```python
from build123d import *

# Parameters (mm, degrees)
SKETCH1_R               = 50
SKETCH1_R_2             = 10
BOSS_EXTRUDE1_DEPTH     = 3
BOSS_EXTRUDE2_DEPTH     = 2.5
CAVITY2_START           = 0.75
CAVITY2_DEPTH           = 2.25
CAVITY2_START_2         = 1.25
CAVITY2_2_DEPTH         = 1.75
FILLET1_R               = 0.5
FILLET2_R               = 7
CUT_EXTRUDE2_DEPTH      = 76.690157881
CUT_EXTRUDE2_DEPTH_BACK = 76.690157881
SKETCH3_R               = 50
SKETCH3_W               = 41.955661048
SKETCH3_H               = 23.335406012


# Read off the part's stored shape, not the designer's step: Cavity2
with BuildPart() as part:
    # Sketch1 → Boss-Extrude1 (new body)
    with BuildSketch(Plane(origin=(0, 0, 0), x_dir=(1, 0, 0), z_dir=(0, 1, 0))):
        with Locations(Location((0, 0, 0), (0, 0, 270))):
            Circle(SKETCH1_R)
        with Locations(Location((0, 0, 0), (0, 0, 270))):
            Circle(SKETCH1_R_2, mode=Mode.SUBTRACT)
    extrude(amount=BOSS_EXTRUDE1_DEPTH)

    # Sketch2 → Boss-Extrude2 (add, symmetric)
    with BuildSketch(Plane.XY.offset(-25)):
        Polygon((-17.5, 3), (-10.5, 3), (-10.5, 23), (30.5, 23), (30.5, 3), (37.5, 3), (37.5, 30), (-17.5, 30), align=None)
    extrude(amount=BOSS_EXTRUDE2_DEPTH, both=True)

    # Cavity2 outline → Cavity2 (cut)
    with BuildSketch(Plane(origin=(0, 0, 0), x_dir=(1, 0, 0), z_dir=(0, 1, 0)).offset(CAVITY2_START)):
        with BuildLine():
            ThreePointArc((-9.944972826, -1.047623734), (-10, 0), (-9.944972826, 1.047623734))
            ThreePointArc((-9.944972826, 1.047623734), (-10.619281402, 1.655282378), (-11.5, 1.875))
            Line((-11.5, 1.875), (-11.5, 8.875))
            Line((-11.5, 8.875), (-24.1, 8.875))
            Line((-24.1, 8.875), (-24.1, -8.875))
            Line((-24.1, -8.875), (-11.5, -8.875))
            Line((-11.5, -8.875), (-11.5, -1.875))
            ThreePointArc((-11.5, -1.875), (-10.619281402, -1.655282378), (-9.944972826, -1.047623734))
        make_face()
    extrude(amount=CAVITY2_DEPTH, mode=Mode.SUBTRACT)

    # Cavity2 2 outline → Cavity2 2 (cut)
    with BuildSketch(Plane(origin=(0, 0, 0), x_dir=(1, 0, 0), z_dir=(0, 1, 0)).offset(CAVITY2_START_2)):
        with BuildLine():
            ThreePointArc((-11.5, 1.875), (-10.619281402, 1.655282378), (-9.944972826, 1.047623734))
            ThreePointArc((-9.944972826, 1.047623734), (-8.262249735, 5.633402996), (-4.608077148, 8.875))
            Line((-4.608077148, 8.875), (-11.5, 8.875))
            Line((-11.5, 8.875), (-11.5, 1.875))
        make_face()
        with BuildLine():
            ThreePointArc((-4.608077148, -8.875), (-8.262249735, -5.633402996), (-9.944972826, -1.047623734))
            ThreePointArc((-9.944972826, -1.047623734), (-10.619281402, -1.655282378), (-11.5, -1.875))
            Line((-11.5, -1.875), (-11.5, -8.875))
            Line((-11.5, -8.875), (-4.608077148, -8.875))
        make_face()
        with BuildLine():
            Line((-24.1, -4.625), (-24.1, 4.625))
            ThreePointArc((-24.1, 4.625), (-26.35, 0), (-24.1, -4.625))
        make_face()
    extrude(amount=CAVITY2_2_DEPTH, mode=Mode.SUBTRACT)

    # Fillet1
    fillet1_edges = [part.edges().sort_by_distance(p)[0] for p in [
        (-14, 3, -22.5),
        (-17.5, 3, -25),
        (34, 3, -27.5),
        (37.5, 3, -25),
        (-14, 3, -27.5),
        (34, 3, -22.5),
    ]]
    fillet(fillet1_edges, radius=FILLET1_R)

    # Fillet2
    fillet2_edges = [part.edges().sort_by_distance(p)[0] for p in [
        (-17.5, 30, -25),
        (37.5, 30, -25),
    ]]
    fillet(fillet2_edges, radius=FILLET2_R)

    # Sketch3 → Cut-Extrude2 (cut, two sides: drawn at the far end of the back side and taken through both)
    with BuildSketch(Plane(origin=(0, 3, 0), x_dir=(1, 0, 0), z_dir=(0, 1, 0)).offset(-CUT_EXTRUDE2_DEPTH_BACK)):
        Circle(SKETCH3_R)
        with Locations((-8.073248433, 0)):
            Rectangle(SKETCH3_W, SKETCH3_H, mode=Mode.SUBTRACT)
    extrude(amount=CUT_EXTRUDE2_DEPTH + CUT_EXTRUDE2_DEPTH_BACK, mode=Mode.SUBTRACT)


solid = part.part
```
Source: CAD feature listing. Evaluate the final solid. Frame: model axes, mm. A direction names the side the tool comes from. Give positions to 0.01 mm unless a question says otherwise; leave off trailing zeros. Write each loop counter-clockwise with the first axis right and the second up, starting at its lowest first coordinate (ties: lowest second). Pieces come first, ordered by that corner, then holes.
1. Access query for faces 4 (the face through (-14, 2, 8.875)), 5 (the face through (-8, 3, -11)). Directions: +Z, -Z, +X, -X, +Y, -Y. A direction counts if a zero-diameter tool reaches every point of the face in a straight line with its end or side. Return the directions, or none.
2. Section query D-D (z = -7.5). Return the cut outline in (x, y).
3. Section query B-B (z = 0). Return the cut outline in (x, y), then the cut area to 3 significant figures.
4. First-contact query: pin 1 (2 mm diameter, centred on x = -8, z = 6.5, fed in from +Y); pin 2 (7 mm diameter, centred on x = -15.5, z = -3, fed in from +Y). Flat tips, straight axial feed; report the tip coordinate or a pass-through.
5. Material intervals for line 1 along X through (y, z) = (2.3, 0); line 2 along X through (y, z) = (0.95, 0); line 3 along Z through (x, y) = (0, 1.2), sorted ascending.
6. Pull-direction query (X, two-part tool) for faces 1 (the face through (12.905, 1, 0)), 2 (the face through (-10, 1.25, 6)), 3 (the face through (-8, 1, -11.668)); classes: +X half, -X half, draft (parallel to the pull), parting line (faces both ways), or undercut.
7. Section query A-A (x = 0). Return the cut outline in (y, z), then the cut area to 3 significant figures.
8. Section query C-C (x = -15.5). Return the cut outline in (y, z) (3 decimals).
Output values:
1. face 4: +Y
1. face 5: +Z, -Z, +X, -X, +Y
2. outline: (-29.05, 0) - (-6.61, 0) - (-6.61, 1.25) - (-11.5, 1.25) - (-11.5, 0.75) - (-24.1, 0.75) - (-24.1, 3) - (-29.05, 3) - close; (6.61, 0) - (12.9, 0) - (12.9, 3) - (6.61, 3) - close
3. outline: (-29.05, 0) - (-10, 0) - (-10, 0.75) - (-24.1, 0.75) - (-24.1, 1.25) - (-26.35, 1.25) - (-26.35, 3) - (-29.05, 3) - close; (10, 0) - (12.9, 0) - (12.9, 3) - (10, 3) - close
3. area: 30.2 mm2
4. pin 1: stops at y = 1.25
4. pin 2: stops at y = 0.75
5. line 1: x = -29.05 to -26.35, 10 to 12.9
5. line 2: x = -29.05 to -24.1, 10 to 12.9
5. line 3: z = -11.67 to -10, 10 to 11.67
6. face 1: +X half
6. face 2: undercut
6. face 3: draft
7. outline: (0, -11.67) - (3, -11.67) - (3, -10) - (0, -10) - close; (0, 10) - (3, 10) - (3, 11.67) - (0, 11.67) - close
7. area: 10.0 mm2
8. outline: (0, -11.668) - (3, -11.668) - (3, -8.875) - (0.75, -8.875) - (0.75, 8.875) - (3, 8.875) - (3, 11.668) - (0, 11.668) - close
